Verification items for the finished model (mm, model axes). Face numbers are marked on the shaded views. A direction names the side the tool comes from. Coordinates: 2 decimals unless noted, no trailing zeros. Loops run counter-clockwise (first coordinate to the right, second up) from the corner with the lowest first, then second, coordinate; pieces in that order, holes last.
Q1. Mould release check, pull along Y, two halves, no side actions. Record for the marked faces 3, 4 and 5: +Y half, -Y half, draft (parallel to the pull), parting line (faces both ways), or undercut.
Q2. Material ranges on probe 1 along Y at (x, z) = (0, -3.25); probe 2 along Y at (x, z) = (0, -14.5); probe 3 along Z at (x, y) = (7.75, -1), recorded low to high.
Q3. Go/stop test with flat-tipped pins: P1, Ø10, axis at y = -3, z = 11.5, coming from the -X side; P2, Ø4, axis at x = 2, y = -1.5, coming from the -Z side; P3, Ø3, axis at y = -3.5, z = 2.5, coming from the +X side; P4, Ø1.5, axis at y = 7, z = 8.5, coming from the -X side. Record where each tip stops, or that it passes through.
Q4. Access from +Z, -Z, +X, -X, +Y, -Y to the whole of each face (thin tool, end or side, straight path). Record for the marked faces 1 and 2.
Q5. Sectioned sample at C-C (z = -9.5). Enter the section's corners in (x, y), then the cut area to 3 significant figures.
```python
from build123d import *

# Parameters (mm, degrees)
F0_R     = 7
F0_R_2   = 3
F1_DEPTH = 20
F0_R_3   = 9.75
F2_DEPTH = 20
F3_R     = 4
F3_R_2   = 3
F4_DEPTH = 10
F5_SIZE  = 0.99999


# Not quite as in the source:
# - a fillet or chamfer is up to 0.001 mm smaller than in the source, because OpenCascade refuses the exact size


with BuildPart() as f1:
    # F0 (on Top) → F1 (new body)
    with BuildSketch(Plane.XY):
        Circle(F0_R)
        Circle(F0_R_2, mode=Mode.SUBTRACT)
    extrude(amount=F1_DEPTH)

    # F0 (on Top) → F2 (join)
    with BuildSketch(Plane.XY):
        Circle(F0_R_3)
        Circle(F0_R, mode=Mode.SUBTRACT)
        Circle(F0_R)
        Circle(F0_R_2, mode=Mode.SUBTRACT)
    extrude(amount=-F2_DEPTH)

    # F3 (on face) → F4 (cut)
    with BuildSketch(Plane(origin=(0, 0, -20), x_dir=(1, 0, 0), z_dir=(0, 0, -1))):
        Circle(F3_R)
        Circle(F3_R_2, mode=Mode.SUBTRACT)
    extrude(amount=-F4_DEPTH, mode=Mode.SUBTRACT)

    # F5 (size 1 in the source; OpenCascade refuses exactly that, so slightly less here)
    f5_edges = [f1.edges().sort_by_distance(p)[0] for p in [
        (-9.75, 0, -20),
        (-7, 0, 20),
        (-3, 0, -10),
    ]]
    chamfer(f5_edges, length=F5_SIZE)


solid = f1.part
```
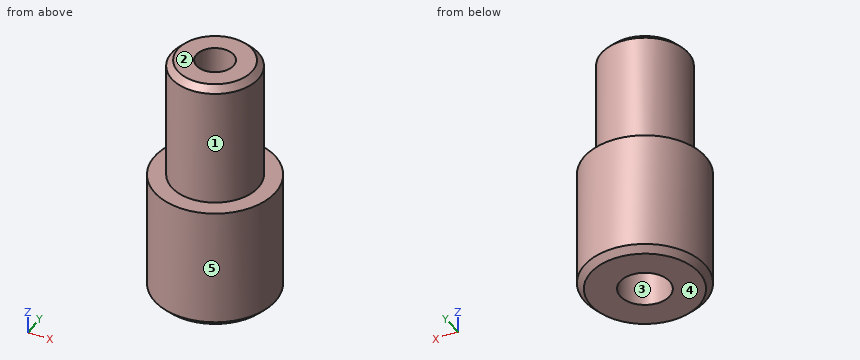
Geometry check:
1. face 3: undercut
1. face 4: draft
1. face 5: parting line
2. probe 1: y = -9.75 to -3, 3 to 9.75
2. probe 2: y = -9.75 to -4, 4 to 9.75
2. probe 3: z = -20 to 0
3. P1: stops at x = -7
3. P2: stops at z = -20
3. P3: stops at x = 6.71
3. P4: stops at x = -3.15
4. face 1: +Z
4. face 2: +Z, +X, -X, +Y, -Y
5. outline: circle Ø19.5 at (0, 0); hole circle Ø7 at (0, 0)
5. area: 260 mm2
